Can you work these out from the drawing? Everything is in mm from the part's minimum corner. Give positions to 0.01 mm unless a question says otherwise; leave off trailing zeros. Order: outer loops, then holes, each group sorted by start corner. A loop starts at its lowest first (then second) coordinate and runs counter-clockwise, first axis right, second up. Notation, with made-up numbers: (19, 55) - (58, 55) arc R27 ccw to (58, 81) - close; hole circle Ø10 at (-14, 58.25). An arc over 180 degrees is marked (long way). One line per question, with ' | ' between items.
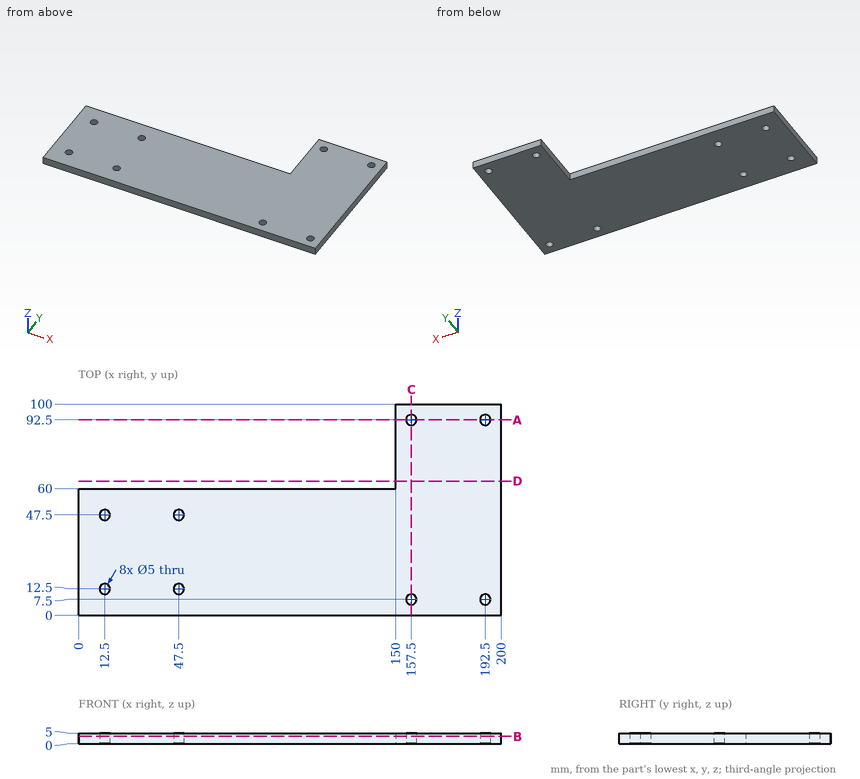
(1) Will these pins go through, and if not, where does the flat tip stop? pin 1 (1.5 mm diameter, centred on y = 73.5, z = 3.5, fed in from -X); pin 2 (4 mm diameter, centred on x = 192.5, y = 92.5, fed in from -Z); pin 3 (2.5 mm diameter, centred on x = 106, z = 1.5, fed in from +Y).
Answer below:
pin 1: x = 150 | pin 2: through | pin 3: y = 60
(2) Imagine slicing it at A-A (y = 92.5). List the corners of the cut face in (x, z) for me.
Answer below:
outline: (150, 0) - (155, 0) - (155, 5) - (150, 5) - close; (160, 0) - (190, 0) - (190, 5) - (160, 5) - close; (195, 0) - (200, 0) - (200, 5) - (195, 5) - close
(3) Imagine slicing it at B-B (z = 3.55). Count the separate pieces of the cut face and the enclosed holes in it, and give its area (3 significant figures).
Answer below:
separate pieces: 1 | enclosed holes: 8 | area: 13,800 mm^2
(4) Imagine slicing it at C-C (x = 157.5). List the corners of the cut face in (y, z) for me.
Answer below:
outline: (0, 0) - (5, 0) - (5, 5) - (0, 5) - close; (10, 0) - (90, 0) - (90, 5) - (10, 5) - close; (95, 0) - (100, 0) - (100, 5) - (95, 5) - close
(5) Imagine slicing it at D-D (y = 63.5). List the corners of the cut face in (x, z) for me, and give its area (3 significant figures).
Answer below:
outline: (150, 0) - (200, 0) - (200, 5) - (150, 5) - close | area: 250 mm^2
(6) If I drill on line 1 (Y direction, x = 12.5, z = 1.1); line 2 (Y direction, x = 157.5, z = 3.4); line 3 (X direction, y = 92.5, z = 3.8), over which ranges is the centre line in solid material (lowest first)?
Answer below:
line 1: 0 to 10, 15 to 45, 50 to 60 | line 2: 0 to 5, 10 to 90, 95 to 100 | line 3: 150 to 155, 160 to 190, 195 to 200
